For this review, take the finished solid that the model builds, in its own axes (mm). A direction names the side the tool comes from. Give positions to 0.01 mm unless a question says otherwise; leave off trailing zeros. Write each loop counter-clockwise with the first axis right and the second up, starting at its lowest first coordinate (ties: lowest second). Pieces come first, ordered by that corner, then holes. Notation, with made-up numbers: (-28, 32.5) -> (19, 32.5) arc R21 cw to (19, 54.5) -> close; hole circle Ø7 at (-35.5, 62). An arc over 180 degrees is marked (long way). Return JSON: item names as keys, results as strings.
from build123d import *

# Parameters (mm, degrees)
F0_R          = 5
F1_DEPTH      = 5
F2_DEPTH      = 15
F3_DEPTH      = 10
F3_DEPTH_BACK = 5


with BuildPart() as f1:
    # F0 (on Front) → F1 (new body)
    with BuildSketch(Plane.XZ):
        with BuildLine():
            Line((35.1758819227, 0), (0, 0))
            ThreePointArc((0, 0), (-10, -10), (0, -20))
            Line((0, -20), (35.1758819227, -20))
            ThreePointArc((35.1758819227, -20), (45.1758819227, -10), (35.1758819227, 0))
        make_face()
        with Locations((0, -10)):
            Circle(F0_R, mode=Mode.SUBTRACT)
        with Locations((35.1758819227, -10)):
            Circle(F0_R, mode=Mode.SUBTRACT)
    extrude(amount=F1_DEPTH)

    # F0 (on Front) → F2 (join)
    with BuildSketch(Plane.XZ):
        with Locations((35.1758819227, -10)):
            Circle(F0_R)
    extrude(amount=F2_DEPTH)

    # F0 (on Front) → F3 (join, two sides)
    with BuildSketch(Plane.XZ) as f3_sk:
        with Locations((0, -10)):
            Circle(F0_R)
    extrude(amount=-F3_DEPTH)
    extrude(f3_sk.sketch, amount=F3_DEPTH_BACK)


solid = f1.part
1. Add section B-B, the plane z = -10. State the section outline as (x, y) points, plus the area to 3 significant figures.
Results found:
{"outline": "(-10, -5) -> (30.18, -5) -> (30.18, -15) -> (40.18, -15) -> (40.18, -5) -> (45.18, -5) -> (45.18, 0) -> (5, 0) -> (5, 10) -> (-5, 10) -> (-5, 0) -> (-10, 0) -> close", "area": "476 mm²"}
2. For faces 1 (the cylindrical face through (-0.651, 4.93, -5.043)), 2 (the cylindrical face through (-10, -2, -10)), 3 (the cylindrical face through (39.8, -9.9, -11.9)), list the 3-axis set-ups (+Z, -Z, +X, -X, +Y, -Y) from which the entire face can be reached by the end or side of a thin tool; tool diameter is ignored.
Results found:
{"face 1": "+Y", "face 2": "-X, +Y, -Y", "face 3": "-Y"}
3. Add section C-C, the plane y = -9. State the section outline as (x, z) points, plus the area to 3 significant figures.
Results found:
{"outline": "circle Ø10 at (35.18, -10)", "area": "78.5 mm²"}
4. Add section D-D, the plane z = -13.5. State the section outline as (x, y) points, plus the area to 3 significant figures.
Results found:
{"outline": "(-9.37, -5) -> (31.61, -5) -> (31.61, -15) -> (38.75, -15) -> (38.75, -5) -> (44.54, -5) -> (44.54, 0) -> (3.57, 0) -> (3.57, 10) -> (-3.57, 10) -> (-3.57, 0) -> (-9.37, 0) -> close", "area": "412 mm²"}
5. Add section A-A, the plane x = 4. State the section outline as (y, z) points, plus the area to 3 significant figures.
Results found:
{"outline": "(-5, -20) -> (0, -20) -> (0, -13) -> (10, -13) -> (10, -7) -> (0, -7) -> (0, 0) -> (-5, 0) -> close", "area": "160 mm²"}
6. For pin 1 (8 mm diameter, centred on x = -4, y = 1.5, fed in from -Z); pin 2 (2 mm diameter, centred on x = 31, y = -8.5, fed in from +Z); pin 3 (6 mm diameter, centred on y = -6, z = -15.5, fed in from -X), all flat-tipped, find the tip position at first contact; note any pin that passes through.
Results found:
{"pin 1": "stops at z = -20", "pin 2": "stops at z = -6.14", "pin 3": "stops at x = -9.64"}
7. To check wall thickness, follow probe 1 along Y at (x, z) = (18, -8); probe 2 along Y at (x, z) = (1.5, -5.5); probe 3 along X at (y, z) = (-13.25, -12.75). State the ranges of each line that lie inside material, in increasing order.
Results found:
{"probe 1": "y = -5 to 0", "probe 2": "y = -5 to 10", "probe 3": "x = 31 to 39.35"}
